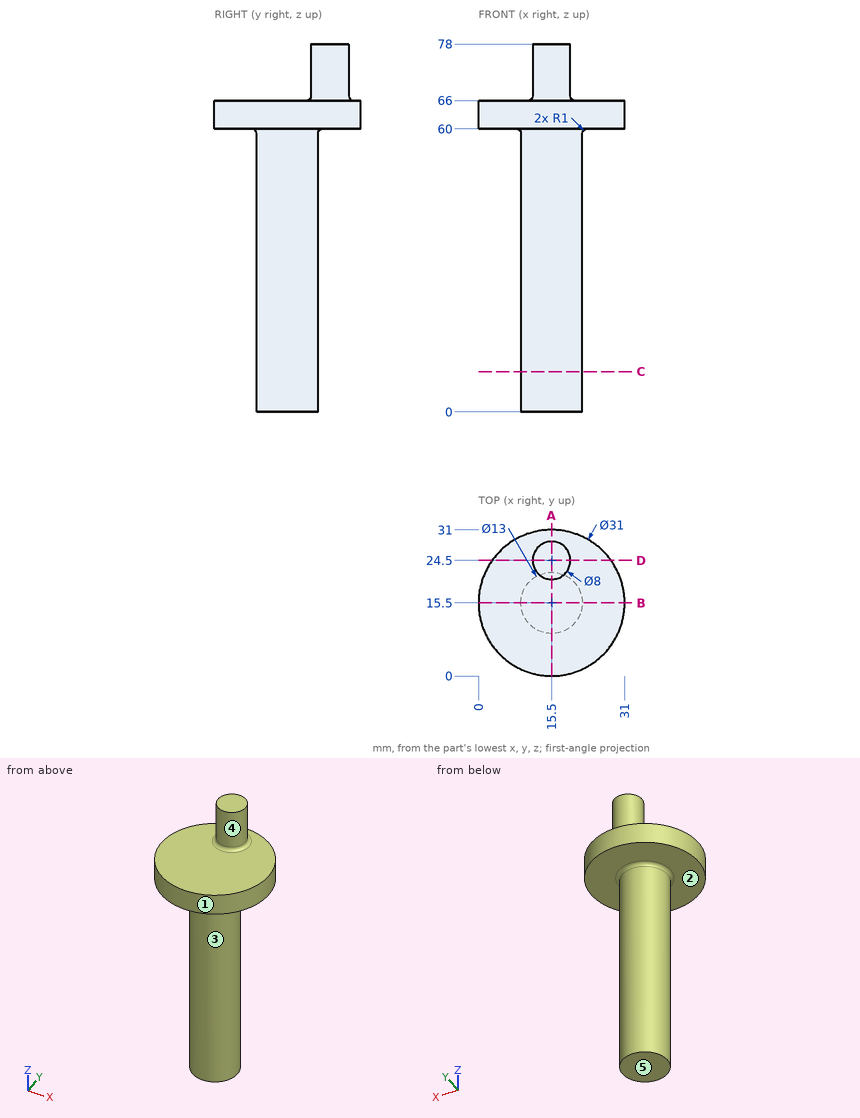
Source: three-view drawing plus pictorial views. Frame: mm from the lowest corner of the part. A direction names the side the tool comes from. Give positions to 0.01 mm unless a question says otherwise; leave off trailing zeros. Loops run counter-clockwise (first coordinate to the right, second up) from the corner with the lowest first, then second, coordinate; pieces in that order, holes last. Notation, with made-up numbers: (59, 86.5) -> (79, 86.5) arc R25 cw to (79, 99.5) -> close; hole circle Ø8 at (4.25, 69). An arc over 180 degrees is marked (long way). Put each result on its own line as item: value. Start each with the question number.
1) Contact query for flat-ended pins moving along their axis: P1, Ø1.5, axis at x = 6, y = 24.5, coming from the -Z side; P2, Ø12, axis at x = 26.5, y = 21.5, coming from the +Z side; P3, Ø15.5, axis at x = 21, y = 18, coming from the +Z side; P4, Ø8, axis at x = 20, z = 64.5, coming from the -Y side. Output: stop coordinate, or through.
2) Reachability of the marked faces 3, 4 and 5 from +Z, -Z, +X, -X, +Y, -Y: full face, straight path, thin tool, end or side. Return the list, or none.
3) Material intervals for probe 1 along Z at (x, y) = (4, 7.5); probe 2 along Z at (x, y) = (16.5, 14.5); probe 3 along Y at (x, z) = (21, 42), sorted ascending.
4) Cut plane A-A (x = 15.5). Return loops of the section in (y, z), then the cut area to 3 significant figures.
5) Cut plane D-D (y = 24.5). Return loops of the section in (x, z), then the cut area to 3 significant figures.
6) Cut plane C-C (z = 8.5). Return loops of the section in (x, y), then the cut area to 3 significant figures.
7) Cut plane B-B (y = 15.5). Return loops of the section in (x, z), then the cut area to 3 significant figures.
8) Draft query along Y for the marked faces 1 and 2. Return one class per face: released by +Y, released by -Y, zero draft, split by the parting line, or undercut.
Results are:
1. P1: stops at z = 60
1. P2: stops at z = 66
1. P3: stops at z = 78
1. P4: stops at y = 0.01
2. face 3: -Z
2. face 4: +Z
2. face 5: -Z, +X, -X, +Y, -Y
3. probe 1: z = 60 to 66
3. probe 2: z = 0 to 66
3. probe 3: y = 12.04 to 18.96
4. outline: (0, 60) -> (8, 60) arc R1 cw to (9, 59) -> (9, 0) -> (22, 0) -> (22, 59) arc R1 cw to (23, 60) -> (31, 60) -> (31, 66) -> (29.5, 66) arc R1 cw to (28.5, 67) -> (28.5, 78) -> (20.5, 78) -> (20.5, 67) arc R1 cw to (19.5, 66) -> (0, 66) -> close
4. area: 1,060 mm2
5. outline: (2.88, 60) -> (28.12, 60) -> (28.12, 66) -> (20.5, 66) arc R1 cw to (19.5, 67) -> (19.5, 78) -> (11.5, 78) -> (11.5, 67) arc R1 cw to (10.5, 66) -> (2.88, 66) -> close
5. area: 248 mm2
6. outline: circle Ø13 at (15.5, 15.5)
6. area: 133 mm2
7. outline: (0, 60) -> (8, 60) arc R1 cw to (9, 59) -> (9, 0) -> (22, 0) -> (22, 59) arc R1 cw to (23, 60) -> (31, 60) -> (31, 66) -> (0, 66) -> close
7. area: 966 mm2
8. face 1: split by the parting line
8. face 2: zero draft
